CAD build for the part. Positions are in the model's coordinates, mm. Face numbers are marked on the shaded views. A direction names the side the tool comes from. Round coordinates to 2 decimals unless told otherwise and drop trailing zeros. Loops run counter-clockwise (first coordinate to the right, second up) from the corner with the lowest first, then second, coordinate; pieces in that order, holes last. Notation, with made-up numbers: M -38.5,49.5 L -2.5,49.5 A11 ccw -2.5,54.5 Z; hole C 58.5,18.25 d6. An arc over 180 degrees is marked long. Use a Markdown table: item, result. Add a question column.
(1) Which spindle directions (+Z, -Z, +X, -X, +Y, -Y) get a long thin tool onto all of the face, cutting with end or side? Do the marked faces 3 and 4. Say none if no direction does.
(2) Band-saw the part on A-A, the plane z = 361. Write the cut outline in (x, y).
(3) Band-saw the part on C-C, the plane y = 122. Write the cut outline in (x, z), and give its area (3 significant figures).
(4) Wall check: L1, parallel to Z at x = 45, y = 47; L2, parallel to X at y = 241.5, z = 426.5; L3, parallel to X at y = -386.5, z = 964.5. Give the ranges that are in metal, low to high.
(5) Two-plate mould, pull along Z, no slides. Class the marked faces 1 and 2: released by +Z, released by -Z, zero draft, split by the parting line, or undercut.
(6) Band-saw the part on D-D, the plane y = 370. Write the cut outline in (x, z).
(7) Band-saw the part on B-B, the plane x = 82.5. Write the cut outline in (y, z), and give its area (3 significant figures).
from build123d import *

# Parameters (mm, degrees)
F0_W     = 914.4
F0_H     = 2438.4
F1_DEPTH = 127
F2_W     = 88.9
F2_H     = 1962.15
F3_DEPTH = 914.4
F5_DEPTH = 2438.401


with BuildPart() as f1:
    # F0 (on Right) → F1 (new body)
    with BuildSketch(Plane.YZ):
        Rectangle(F0_W, F0_H)
    extrude(amount=F1_DEPTH)

    # F2 (on face) → F3 (cut, through all)
    with BuildSketch(Plane.XZ.offset(457.2)):
        with Locations((63.5, 219.075)):
            Rectangle(F2_W, F2_H)
    extrude(amount=-F3_DEPTH, mode=Mode.SUBTRACT)

    # F4 (on face) → F5 (cut, through all)
    with BuildSketch(Plane.XY.offset(1219.2)):
        Polygon((0, 304.8), (127, 457.2), (0, 457.2), align=None)
        Polygon((127, -457.2), (127, -304.8), (0, -457.2), align=None)
    extrude(amount=-F5_DEPTH, mode=Mode.SUBTRACT)


solid = f1.part
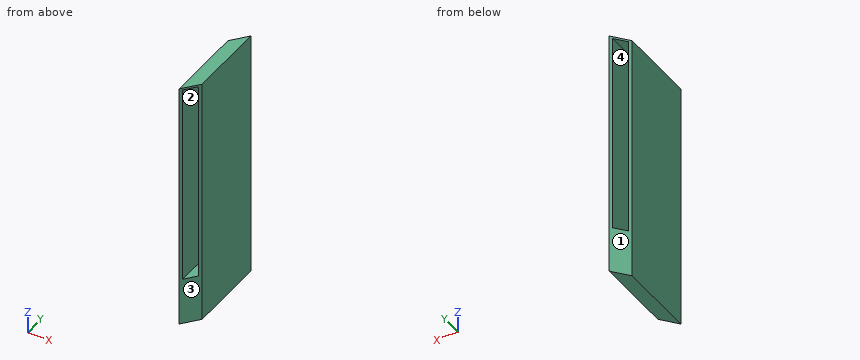
Return value:
| question | item | result |
|---|---|---|
| 1 | face 3 | +Z, -Z, +X, -Y |
| 1 | face 4 | +Y, -Y |
| 2 | outline | M 0,-457.2 L 19.05,-434.34 L 19.05,327.66 L 0,304.8 Z; M 107.95,-327.66 L 127,-304.8 L 127,457.2 L 107.95,434.34 Z |
| 3 | outline | M 0,-1219.2 L 127,-1219.2 L 127,1219.2 L 0,1219.2 Z; hole M 19.05,-762 L 107.95,-762 L 107.95,1200.15 L 19.05,1200.15 Z |
| 3 | area | 135,000 mm^2 |
| 4 | L1 | -1219.2 to -762, 1200.15 to 1219.2 |
| 4 | L2 | 0 to 19.05, 107.95 to 127 |
| 4 | L3 | 0 to 19.05 |
| 5 | face 1 | zero draft |
| 5 | face 2 | undercut |
| 6 | outline | M 54.33,-1219.2 L 127,-1219.2 L 127,1219.2 L 54.33,1219.2 L 54.33,1200.15 L 107.95,1200.15 L 107.95,-762 L 54.33,-762 Z |
| 7 | outline | M -358.2,-1219.2 L 403.8,-1219.2 L 403.8,-762 L -358.2,-762 Z; M -358.2,1200.15 L 403.8,1200.15 L 403.8,1219.2 L -358.2,1219.2 Z |
| 7 | area | 363,000 mm^2 |
